Verification items for the finished model (mm, model axes). Round coordinates to 2 decimals unless told otherwise and drop trailing zeros. Loops run counter-clockwise (first coordinate to the right, second up) from the corner with the lowest first, then second, coordinate; pieces in that order, holes last. Notation, with made-up numbers: (79.25, 0) -> (99.25, 0) arc R22 cw to (99.25, 7) -> close; hole circle Ø9 at (28.5, 34.5). An arc over 180 degrees is marked (long way). Use a Markdown table: item, result. Add a question column.
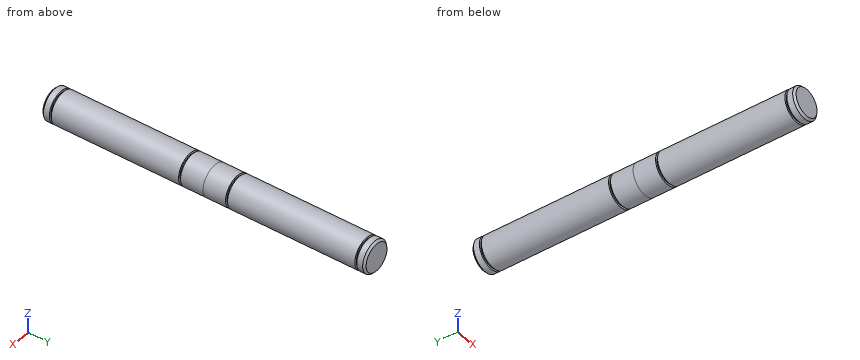
```python
from build123d import *

# Parameters (mm, degrees)
CHAMFER1_SIZE = 1


with BuildPart() as part:
    # Sketch2 → Revolve1 (revolve)
    with BuildSketch(Plane.XY, mode=Mode.PRIVATE) as revolve1_sk:
        Polygon((0, 0), (8, 0), (8, 11.5), (7, 11.5), (7, 12.5), (8, 12.5), (8, 77.5), (7, 77.5), (7, 78.5), (8, 78.5), (8, 82.5), (0, 82.5), align=None)
    revolve1 = revolve(revolve1_sk.sketch.rotate(Axis((0, 82.5, 0), (0, -1, 0)), 180), axis=Axis((0, 82.5, 0), (0, -1, 0)))

    # Mirror1: Revolve1 across plane
    add(revolve1.mirror(Plane.ZX))

    # Chamfer1
    chamfer1_edges = [part.edges().sort_by_distance(p)[0] for p in [
        (8, -82.5, 0),
        (8, 82.5, 0),
    ]]
    chamfer(chamfer1_edges, length=CHAMFER1_SIZE)


solid = part.part
```
1) Go/stop test with flat-tipped pins: pin 1 (2 mm diameter, centred on y = 63, z = 5, fed in from +X); pin 2 (6 mm diameter, centred on x = 6.5, y = 7, fed in from +Z); pin 3 (1 mm diameter, centred on x = -6, z = 5.5, fed in from -Y). Record where each tip stops, or that it passes through.
2) Thickness scan on line 1 (X direction, y = 39, z = -0.5); line 2 (Y direction, x = -3.25, z = 6.75); line 3 (Z direction, x = 0.25, y = -21). Record the ranges inside material, lowest first.
3) Sectioned sample at A-A on y = -33.5. Enter the section's corners in (x, z), then the cut area to 3 significant figures.
Geometry results:
| question | item | result |
|---|---|---|
| 1 | pin 1 | x = 6.93 |
| 1 | pin 2 | z = 7.19 |
| 1 | pin 3 | y = -81.86 |
| 2 | line 1 | -7.98 to 7.98 |
| 2 | line 2 | -82.01 to -78.5, -77.5 to -12.5, -11.5 to 11.5, 12.5 to 77.5, 78.5 to 82.01 |
| 2 | line 3 | -8 to 8 |
| 3 | outline | circle Ø16 at (0, 0) |
| 3 | area | 201 mm^2 |
